Answer from the drawing. Dimensions are ordinates in mm from the lowest x, y and z of the part. Coordinates: 2 decimals unless noted, no trailing zeros. Order: outer loops, then holes, each group sorted by start corner. A loop starts at its lowest first (then second) coordinate and runs counter-clockwise, first axis right, second up.
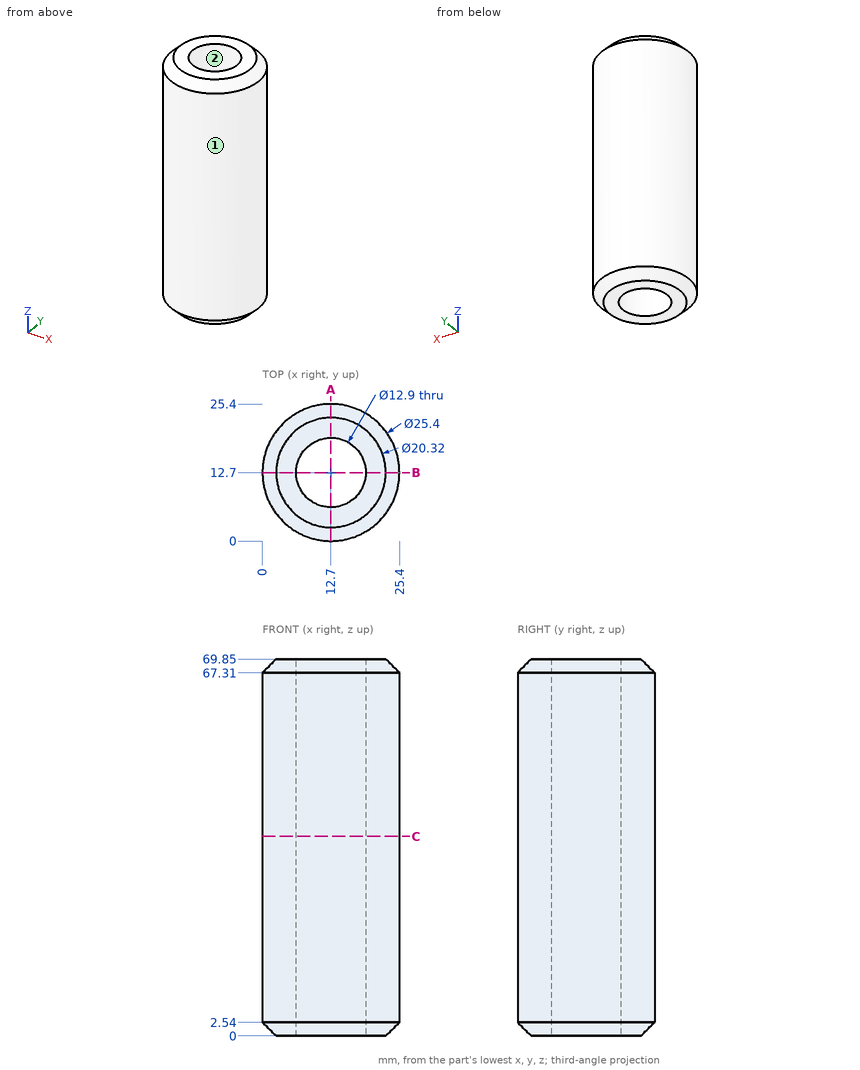
1) Each of these flat-tipped pins is pushed along its axis until it touches: P1, Ø1, axis at x = 3.5, z = 34.5, coming from the +Y side; P2, Ø12, axis at y = 6, z = 54.5, coming from the -X side; P3, Ø1.5, axis at y = 5, z = 15, coming from the +X side. Where does it stop, or does it pass through?
2) Consider L1, parallel to Y at x = 12.7, z = 49.5; L2, parallel to X at y = 8.25, z = 6.5; L3, parallel to X at y = 7, z = 5. Determine where each line is inside the solid, lowest interval first.
3) Section C-C (z = 37) is taken. Give the vertices of the cut face in (x, y), then the cut area to 3 significant figures.
4) Determine the mould class of the marked faces 1 and 2 for opening direction X: released by +X, released by -X, zero draft, split by the parting line, or undercut.
5) Section A-A (x = 12.7) is taken. Give the vertices of the cut face in (y, z).
Filled sheet:
1. P1: stops at y = 21.95
1. P2: stops at x = 0.02
1. P3: stops at x = 23.33
2. L1: y = 0 to 6.25, 19.15 to 25.4
2. L2: x = 0.81 to 8.03, 17.37 to 24.59
2. L3: x = 1.35 to 9.68, 15.72 to 24.05
3. outline: circle Ø25.4 at (12.7, 12.7); hole circle Ø12.9 at (12.7, 12.7)
3. area: 376 mm2
4. face 1: split by the parting line
4. face 2: undercut
5. outline: (0, 2.54) - (2.54, 0) - (6.25, 0) - (6.25, 69.85) - (2.54, 69.85) - (0, 67.31) - close; (19.15, 0) - (22.86, 0) - (25.4, 2.54) - (25.4, 67.31) - (22.86, 69.85) - (19.15, 69.85) - close
